Design review of the part built by this model. Coordinates are the model's own, in mm. Give positions to 0.01 mm unless a question says otherwise; leave off trailing zeros. Loops run counter-clockwise (first coordinate to the right, second up) from the corner with the lowest first, then second, coordinate; pieces in that order, holes last. Notation, with made-up numbers: (54.5, -27) -> (71.5, -27) arc R28 cw to (71.5, -5) -> close; hole circle Ø9 at (69.5, 25). An arc over 180 degrees is marked (long way). Use a Markdown table: item, result. Add a question column.
1. To check wall thickness, follow line 1 (Y direction, x = 158.5, z = 4.5); line 2 (Y direction, x = 126, z = 7.75); line 3 (Z direction, x = 96, y = 217.5). State the ranges of each line that lie inside material, in increasing order.
2. Add section D-D (z = 6.5). Count the separate pieces of the cut face and the enclosed holes in it, and give its area (3 significant figures).
3. Add section B-B (y = 169). State the section outline as (x, z) points, and give its area (3 significant figures).
4. Add section C-C (x = 143.5). State the section outline as (y, z) points, and give its area (3 significant figures).
5. For pin 1 Ø4 at (x, z) = (128, 4.5) entering from -Y; pin 2 Ø1 at (y, z) = (163, 6) entering from +X; pin 3 Ø1.5 at (y, z) = (36.5, 9) entering from -X, all flat-tipped, find the tip position at first contact; note any pin that passes through.
6. Add section A-A (x = 99). State the section outline as (y, z) points, and give its area (3 significant figures).
```python
from build123d import *

# Parameters (mm, degrees)
PAD_DEPTH              = 6.25
FILLET_R               = 6.4
MIRROR_ROLL_ANGLE      = -179.860361
MIRROR_PITCH_ANGLE     = 0.86933
MIRROR_PLACEMENT_ANGLE = 0.335531


with BuildPart() as body:
    # Sketch → Pad (new body)
    with BuildSketch(Plane.XY):
        Polygon((0, 250), (50, 250), (150, 0), (120, 0), (120, 13.2), (30, 13.2), (30, 0), (0, 0), align=None)
        Polygon((15, 230), (15, 135), (79.844506, 135), (41.844506, 230), align=None, mode=Mode.SUBTRACT)
        Polygon((15, 115), (15, 33.2), (120.564506, 33.2), (87.844506, 115), align=None, mode=Mode.SUBTRACT)
        with BuildLine():
            ThreePointArc((18, 243.25), (14.75, 240), (18, 236.75))
            Line((18, 236.75), (38, 236.75))
            ThreePointArc((38, 236.75), (41.25, 240), (38, 243.25))
            Line((38, 243.25), (18, 243.25))
        make_face(mode=Mode.SUBTRACT)
        with BuildLine():
            ThreePointArc((60.5, 128.25), (57.25, 125), (60.5, 121.75))
            Line((60.5, 121.75), (80.5, 121.75))
            ThreePointArc((80.5, 121.75), (83.75, 125), (80.5, 128.25))
            Line((80.5, 128.25), (60.5, 128.25))
        make_face(mode=Mode.SUBTRACT)
        with BuildLine():
            ThreePointArc((18, 128.25), (14.75, 125), (18, 121.75))
            Line((18, 121.75), (38, 121.75))
            ThreePointArc((38, 121.75), (41.25, 125), (38, 128.25))
            Line((38, 128.25), (18, 128.25))
        make_face(mode=Mode.SUBTRACT)
        with BuildLine():
            ThreePointArc((18, 26.45), (14.75, 23.2), (18, 19.95))
            Line((18, 19.95), (38, 19.95))
            ThreePointArc((38, 19.95), (41.25, 23.2), (38, 26.45))
            Line((38, 26.45), (18, 26.45))
        make_face(mode=Mode.SUBTRACT)
        with BuildLine():
            ThreePointArc((101, 26.45), (97.75, 23.2), (101, 19.95))
            Line((101, 19.95), (121, 19.95))
            ThreePointArc((121, 19.95), (124.25, 23.2), (121, 26.45))
            Line((121, 26.45), (101, 26.45))
        make_face(mode=Mode.SUBTRACT)
    extrude(amount=PAD_DEPTH)

    # Fillet
    fillet_edges = [body.edges().sort_by_distance(p)[0] for p in [
        (0, 0, 3.125),
        (50, 250, 3.125),
        (0, 250, 3.125),
        (150, 0, 3.125),
        (120, 0, 3.125),
        (30, 0, 3.125),
        (41.844506, 230, 3.125),
        (15, 230, 3.125),
        (87.844506, 115, 3.125),
        (15, 115, 3.125),
        (15, 135, 3.125),
        (15, 33.2, 3.125),
        (120.564506, 33.2, 3.125),
        (79.844506, 135, 3.125),
        (30, 13.2, 3.125),
        (120, 13.2, 3.125),
    ]]
    fillet(fillet_edges, radius=FILLET_R)


with BuildPart() as model_body_mirrored:
    # mirror: instance of Body
    add(body.part.mirror(Plane(origin=(159.181488, 124.226166, 5.790833), x_dir=(-0.001618, 0.999999, 0), z_dir=(-0.999887, -0.001617, 0.014919))))


with BuildPart() as model_body_mirrored_1:
    # mirror roll: moved
    add(model_body_mirrored.part.rotate(Axis((0, 0, 0), (1, 0, 0)), MIRROR_ROLL_ANGLE))


with BuildPart() as model_body_mirrored_2:
    # mirror pitch: moved
    add(model_body_mirrored_1.part.rotate(Axis((0, 0, 0), (0, 1, 0)), MIRROR_PITCH_ANGLE))


with BuildPart() as model_body_mirrored_3:
    # mirror placement: moved
    add(model_body_mirrored_2.part.moved(Location((-110.969424, 247.905415, 10.458181))).rotate(Axis((-110.969424, 247.905415, 10.458181), (0, 0, 1)), MIRROR_PLACEMENT_ANGLE))


solid = model_body_mirrored_3.part
```
Taken from the geometry:
| question | item | result |
|---|---|---|
| 1 | line 1 | y = 0.64 to 38.77, 114.13 to 134.13, 215.93 to 235.93 |
| 1 | line 2 | y = 79.16 to 121.13, 126.96 to 134.04, 215.84 to 235.84 |
| 1 | line 3 | z = 2.41 to 8.66 |
| 2 | separate pieces | 1 |
| 2 | enclosed holes | 7 |
| 2 | area | 11,400 mm^2 |
| 3 | outline | (89.78, 8.45) -> (89.88, 2.2) -> (106.05, 2.44) -> (105.95, 8.69) -> close; (192.79, 9.96) -> (192.88, 3.71) -> (207.88, 3.93) -> (207.79, 10.18) -> close |
| 3 | area | 195 mm^2 |
| 4 | outline | (35.69, 8.91) -> (35.93, 2.66) -> (76.06, 2.76) -> (75.82, 9.01) -> close; (114.08, 9.1) -> (114.1, 2.85) -> (120.85, 2.87) -> (120.83, 9.12) -> close; (127.33, 9.14) -> (127.35, 2.88) -> (134.1, 2.9) -> (134.08, 9.15) -> close; (215.88, 9.35) -> (215.9, 3.1) -> (235.9, 3.15) -> (235.88, 9.4) -> close |
| 4 | area | 460 mm^2 |
| 5 | pin 1 | stops at y = 69.36 |
| 5 | pin 2 | stops at x = 207.88 |
| 5 | pin 3 | stops at x = 142.87 |
| 6 | outline | (146.12, 8.53) -> (146.36, 2.28) -> (186.49, 2.38) -> (186.25, 8.63) -> close; (215.77, 8.7) -> (215.78, 2.45) -> (222.53, 2.47) -> (222.52, 8.72) -> close; (229.02, 8.74) -> (229.03, 2.48) -> (235.78, 2.5) -> (235.77, 8.75) -> close |
| 6 | area | 335 mm^2 |
